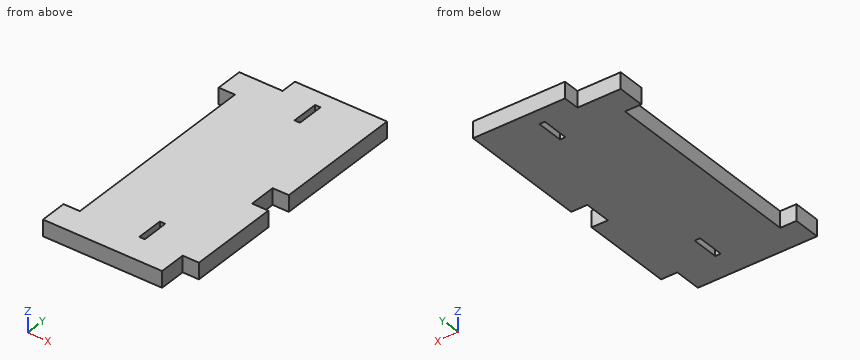
Autodesk Inventor part; units mm, degrees
ref_plane "YZ Plane" through (0, 0, 0) normal (1, 0, 0) x (0, 1, 0)
ref_plane "XZ Plane" through (0, 0, 0) normal (0, 1, 0) x (-1, 0, 0)
ref_plane "XY Plane" through (0, 0, 0) normal (0, 0, 1) x (1, 0, 0)
sketch "Sketch1" plane through (0, 0, 0) normal (0, 0, 1) x (1, 0, 0)
  line L0 (-3, 4.65) -> (-3, 21.525)
  line L1 (0, 4.65) -> (-3, 4.65)
  line L2 (0, 21.525) -> (0, 4.65)
  line L3 (0, 21.525) -> (-3, 21.525)
  line L4 (-3, -0.35) -> (-3, 4.65)
  line L5 (-3, -0.35) -> (-22, -0.35)
  line L6 (-3, 21.525) -> (-3, 26.525)
  line L7 (-3, 26.525) -> (-3, 47.4)
  line L8 (0, 26.525) -> (-3, 26.525)
  line L9 (0, 47.4) -> (0, 26.525)
  line L10 (0, 47.4) -> (-3, 47.4)
  line L11 (-10, 47.4) -> (-10, 42.4)
  line L12 (-11, 47.4) -> (-10, 47.4)
  line L13 (-11, 42.4) -> (-11, 47.4)
  line L14 (-11, 42.4) -> (-10, 42.4)
  line L15 (-10, 9.65) -> (-10, 4.65)
  line L16 (-11, 9.65) -> (-10, 9.65)
  line L17 (-11, 4.65) -> (-11, 9.65)
  line L18 (-11, 4.65) -> (-10, 4.65)
  line L19 (0, 47.4) -> (0, 50.4)
  line L20 (0, 50.4) -> (-22, 50.4)
  line L21 (-22, 50.4) -> (-22, -0.35)
  line L22 (-22, -0.35) -> (-25, -0.35)
  line L23 (-25, -0.35) -> (-25, 4.65)
  line L24 (-25, 4.65) -> (-22, 4.65)
  line L25 (-22, 4.65) -> (-22, -0.35)
  line L26 (-22, 47.4) -> (-25, 47.4)
  line L27 (-25, 47.4) -> (-25, 42.4)
  line L28 (-25, 42.4) -> (-22, 42.4)
  line L29 (-22, 42.4) -> (-22, 47.4)
  line L30 (-22, 50.4) -> (-17, 50.4)
  line L31 (-17, 50.4) -> (-17, 47.4)
  line L32 (-17, 47.4) -> (-22, 47.4)
  line L33 (-22, 47.4) -> (-22, 50.4)
  line L34 (-25, -0.35) -> (-25, -5.35)
  point P0 (0, 0)
extrude "Extrusion1" add sketch "Sketch1" along normal blind 3 contours L4 L5 L21 L32 L31 L20 L19 L10 L7 L6 L0 | L0 L3 L2 L1 | L7 L10 L9 L8 | L22 L23 L24 L21 | L28 L27 L26 L21
properties part number "SideLeftLower" material "Acrylic, Clear"
Check sheet for the modelled part. Datum: model origin and axes. Units: mm. Round coordinates to 2 decimals unless told otherwise and drop trailing zeros. Order: outer loops, then holes, each group sorted by start corner. A loop starts at its lowest first (then second) coordinate and runs counter-clockwise, first axis right, second up. Notation, with made-up numbers: M -6.75,27 L 40.25,27 A18 ccw 40.25,50 Z; hole C -14,-31.5 d4. An arc over 180 degrees is marked long. Answer in a Markdown table with one row per item.
(1) Gauge pin test, flat ends, axial feed: pin 1 (1.5 mm diameter, centred on x = -21.5, z = 1.5, fed in from +Y); pin 2 (1.5 mm diameter, centred on y = 6.5, z = 1.5, fed in from +X); pin 3 (0.9 mm diameter, centred on y = 3, z = 2, fed in from +X); pin 4 (0.9 mm diameter, centred on x = -1, z = 2, fed in from -Y). Record the tip position at first contact, or that the pin passes through.
Findings:
| item | result |
|---|---|
| pin 1 | stops at y = 47.4 |
| pin 2 | stops at x = 0 |
| pin 3 | stops at x = -3 |
| pin 4 | stops at y = 4.65 |
(2) Section check B-B on z = 2.5. Record the boundary of the cut face in (x, y) (3 decimals), plus the area to 3 significant figures.
Findings:
| item | result |
|---|---|
| outline | M -25,-0.35 L -3,-0.35 L -3,4.65 L 0,4.65 L 0,21.525 L -3,21.525 L -3,26.525 L 0,26.525 L 0,50.4 L -17,50.4 L -17,47.4 L -25,47.4 L -25,42.4 L -22,42.4 L -22,4.65 L -25,4.65 Z; hole M -11,4.65 L -10,4.65 L -10,9.65 L -11,9.65 Z; hole M -11,42.4 L -10,42.4 L -10,47.4 L -11,47.4 Z |
| area | 1,090 mm^2 |
(3) Material ranges on line 1 along Y through (x, z) = (-10.25, 2.3); line 2 along X through (y, z) = (8.5, 0.75); line 3 along X through (y, z) = (39, 1.35), recorded low to high. Write a range as from..to.
Findings:
| item | result |
|---|---|
| line 1 | y = -0.35..4.65, 9.65..42.4, 47.4..50.4 |
| line 2 | x = -22..-11, -10..0 |
| line 3 | x = -22..0 |
(4) Section check C-C on y = 15.5. Record the boundary of the cut face in (x, z).
Findings:
| item | result |
|---|---|
| outline | M -22,0 L 0,0 L 0,3 L -22,3 Z |
(5) Section check A-A on x = -2.5. Record the boundary of the cut face in (y, z) (3 decimals).
Findings:
| item | result |
|---|---|
| outline | M 4.65,0 L 21.525,0 L 21.525,3 L 4.65,3 Z; M 26.525,0 L 50.4,0 L 50.4,3 L 26.525,3 Z |
